For this review, take the finished solid that the model builds, in its own axes (mm). A direction names the side the tool comes from. Round coordinates to 2 decimals unless told otherwise and drop trailing zeros. Loops run counter-clockwise (first coordinate to the right, second up) from the corner with the lowest first, then second, coordinate; pieces in that order, holes last.
1) Take a section at B-B (x = -14). State the section outline as (y, z) points (3 decimals).
2) Tool access review of faces 1 (the flat face through (-13, 0, 102)), 2 (the flat face through (-14, 3.175, 100)): name each direction out of +Z, -Z, +X, -X, +Y, -Y from which nothing blocks a thin tool from reaching the whole face with its end or side.
3) Wall thickness on L1, parallel to X at y = 2.5, z = 114.3 (3 decimals); L2, parallel to X at y = 12.5, z = 122.5 (3 decimals); L3, parallel to Y at x = -10, z = 134 (3 decimals): over which ranges is each line inside the solid? List them lowest first.
4) Take a section at A-A (z = 114.3). State the section outline as (x, y) points (3 decimals), then the cut area to 3 significant figures.
5) Insertion check: pin 1 (12 mm diameter, centred on y = 16, z = 104.5, fed in from -X) (3 decimals); pin 2 (10 mm diameter, centred on x = -18, y = 11.5, fed in from +Z); pin 3 (1.5 mm diameter, centred on x = -18, z = 39.5, fed in from +Y) (3 decimals). Each pin has a flat end and moves straight along its axis. Give the tip position at first contact, or say it passes through.
6) Take a section at C-C (z = 147.5). State the section outline as (x, y) points (3 decimals), then the cut area to 3 significant figures.
7) Take a section at D-D (y = 5.25). State the section outline as (x, z) points (3 decimals), then the cut area to 3 significant figures.
8) Mouldability with a two-part tool opening along Z and no side actions: class faces 3 (the flat face through (-7, 2, 0)), 4 (the cylindrical face through (-13.39, 1.61, 117.4)), 5 (the flat face through (-6.996, 2.293, 199.379)), 6 (the flat face through (-25.4, 2, 89)) as pulls with the +Z half, pulls with the -Z half, needs draft (parallel to the pull), parting line crosses it, or undercut.
Autodesk Inventor part; units mm, degrees
ref_plane "YZ Plane" through (0, 0, 0) normal (1, 0, 0) x (0, 1, 0)
ref_plane "XZ Plane" through (0, 0, 0) normal (0, 1, 0) x (-1, 0, 0)
ref_plane "XY Plane" through (0, 0, 0) normal (0, 0, 1) x (1, 0, 0)
sketch "Sketch1" plane through (0, 0, 0) normal (0, 0, 1) x (1, 0, 0)
  line L0 (-25.4, 3.175) -> (-3.175, 3.175)
  line L1 (0, 0) -> (-25.4, 0)
  line L2 (-25.4, 0) -> (-25.4, 3.175)
  line L3 (-3.175, 3.175) -> (-3.175, 25.4)
  line L4 (-3.175, 25.4) -> (0, 25.4)
  line L5 (0, 25.4) -> (0, 0)
  dimension "d0" = 25.4
  dimension "d1" = 25.4
  dimension "d2" = 3.175
  dimension "d3" = 3.175
extrude "Extrusion1" add sketch "Sketch1" along normal blind 206.375
sketch "Sketch2" plane through (-25.4, 0, 0) normal (0, -1, 0) x (1, 0, 0)
  line L0 (25.4, 206.375) -> (0, 206.375)
  line L1 (0, 0) -> (0, 206.375)
  line L2 (25.4, 0) -> (25.4, 206.375)
  line L3 (25.4, 206.375) -> (0, 180.975)
  dimension "d6" = 45
extrude "Extrusion2" cut sketch "Sketch2" against normal blind 177.8
sketch "Sketch3" plane through (-25.4, 3.175, 0) normal (0, 1, 0) x (1, 0, 0)
  line L0 (22.225, 0) -> (22.225, -203.2)
  line L1 (0, 0) -> (22.225, 0)
  circle A0 centre (12.7, -114.3) radius 3.175
  point P0 (25.4, 0)
  dimension "d9" = 6.35
  dimension "d10" = 114.3
  dimension "d11" = 9.525
extrude "Extrusion3" cut sketch "Sketch3" against normal blind 25.4
properties part number "L frame"
Response:
1. outline: (0, 0) - (3.175, 0) - (3.175, 111.403) - (0, 111.403) - close; (0, 117.197) - (3.175, 117.197) - (3.175, 192.375) - (0, 192.375) - close
2. face 1: +Z, -Z, +X, -X, -Y
2. face 2: +Z, -Z, -X, +Y
3. L1: x = -25.4 to -15.875, -9.525 to 0
3. L2: x = -3.175 to 0
3. L3: y = 0 to 3.175
4. outline: (-25.4, 0) - (-15.875, 0) - (-15.875, 3.175) - (-25.4, 3.175) - close; (-9.525, 0) - (0, 0) - (0, 25.4) - (-3.175, 25.4) - (-3.175, 3.175) - (-9.525, 3.175) - close
4. area: 131 mm2
5. pin 1: stops at x = -3.175
5. pin 2: passes through
5. pin 3: stops at y = 3.175
6. outline: (-25.4, 0) - (0, 0) - (0, 25.4) - (-3.175, 25.4) - (-3.175, 3.175) - (-25.4, 3.175) - close
6. area: 151 mm2
7. outline: (-3.175, 0) - (0, 0) - (0, 206.375) - (-3.175, 203.2) - close
7. area: 650 mm2
8. face 3: pulls with the -Z half
8. face 4: undercut
8. face 5: pulls with the +Z half
8. face 6: needs draft
